Check sheet for the modelled part. Datum: model origin and axes. Units: mm. Round coordinates to 2 decimals unless told otherwise and drop trailing zeros. Loops run counter-clockwise (first coordinate to the right, second up) from the corner with the lowest first, then second, coordinate; pieces in that order, holes last. Notation, with made-up numbers: (-5, 82.5) - (16, 82.5) arc R21 ccw to (16, 119.5) - close; hole circle Ø5 at (-31, -23.75). An arc over 180 degrees is marked (long way). Put each result on its own line as item: value.
```python
from build123d import *

# Parameters (mm, degrees)
SKETCH1_W          = 7.5
SKETCH1_H          = 189
SKETCH2_W          = 3
SKETCH2_H          = 3
CUT_EXTRUDE1_DEPTH = 18
SKETCH3_W          = 3
SKETCH3_H          = 3
CUT_EXTRUDE2_DEPTH = 15
CHAMFER1_SIZE      = 1


with BuildPart() as part:
    # Sketch1 → Revolve1 (revolve)
    with BuildSketch(Plane.XY, mode=Mode.PRIVATE) as revolve1_sk:
        with Locations((3.75, 94.5)):
            Rectangle(SKETCH1_W, SKETCH1_H)
    revolve(revolve1_sk.sketch.rotate(Axis((0, 189, 0), (0, -1, 0)), 180), axis=Axis((0, 189, 0), (0, -1, 0)))

    # Sketch2 → Cut-Extrude1 (cut)
    with BuildSketch(Plane(origin=(0, 169, 0), x_dir=(1, 0, 0), z_dir=(0, 1, 0))):
        with Locations((0, 7.5)):
            Rectangle(SKETCH2_W, SKETCH2_H)
    extrude(amount=-CUT_EXTRUDE1_DEPTH, mode=Mode.SUBTRACT)

    # Sketch3 → Cut-Extrude2 (cut)
    with BuildSketch(Plane(origin=(0, 104, 0), x_dir=(-1, 0, 0), z_dir=(0, -1, 0))):
        with Locations((0, 7.5)):
            Rectangle(SKETCH3_W, SKETCH3_H)
    extrude(amount=CUT_EXTRUDE2_DEPTH, mode=Mode.SUBTRACT)

    # Chamfer1
    chamfer1_edges = [part.edges().sort_by_distance(p)[0] for p in [
        (7.5, 0, 0),
        (7.5, 189, 0),
    ]]
    chamfer(chamfer1_edges, length=CHAMFER1_SIZE)


solid = part.part
```
Item 1: Thickness scan on line 1 (Z direction, x = 0.75, y = 22.5); line 2 (X direction, y = 175.5, z = -2.25); line 3 (Z direction, x = 1.5, y = 31.5). Record the ranges inside material, lowest first. Write a range as from..to.
Filled sheet:
line 1: -7.46..7.46
line 2: -7.15..7.15
line 3: -7.35..7.35
Item 2: Release check for a two-part mould opening along X. For faces 1 (the flat face through (0, 160, -6)), 2 (the flat face through (0, 189, 0)), 3 (the flat face through (0, 97, -6)), 4 (the cylindrical face through (1.63, 95.81, 7.32)) record: +X half, -X half, draft (parallel to the pull), parting line (faces both ways), or undercut.
Filled sheet:
face 1: undercut
face 2: draft
face 3: undercut
face 4: parting line
Item 3: Go/stop test with flat-tipped pins: pin 1 (5 mm diameter, centred on x = -4, z = 2, fed in from -Y); pin 2 (1.5 mm diameter, centred on y = 164, z = -6.5, fed in from +X); pin 3 (0.8 mm diameter, centred on x = 0.5, z = -7, fed in from -Y); pin 4 (1.5 mm diameter, centred on x = 0.5, y = 98.5, fed in from -Z). Record where each tip stops, or that it passes through.
Filled sheet:
pin 1: y = 0
pin 2: x = 4.82
pin 3: y = 0.12
pin 4: z = -6
Item 4: Section check A-A on y = 106.5. Enter the section's corners in (x, z), then the cut area to 3 significant figures.
Filled sheet:
outline: circle Ø15 at (0, 0)
area: 177 mm²
